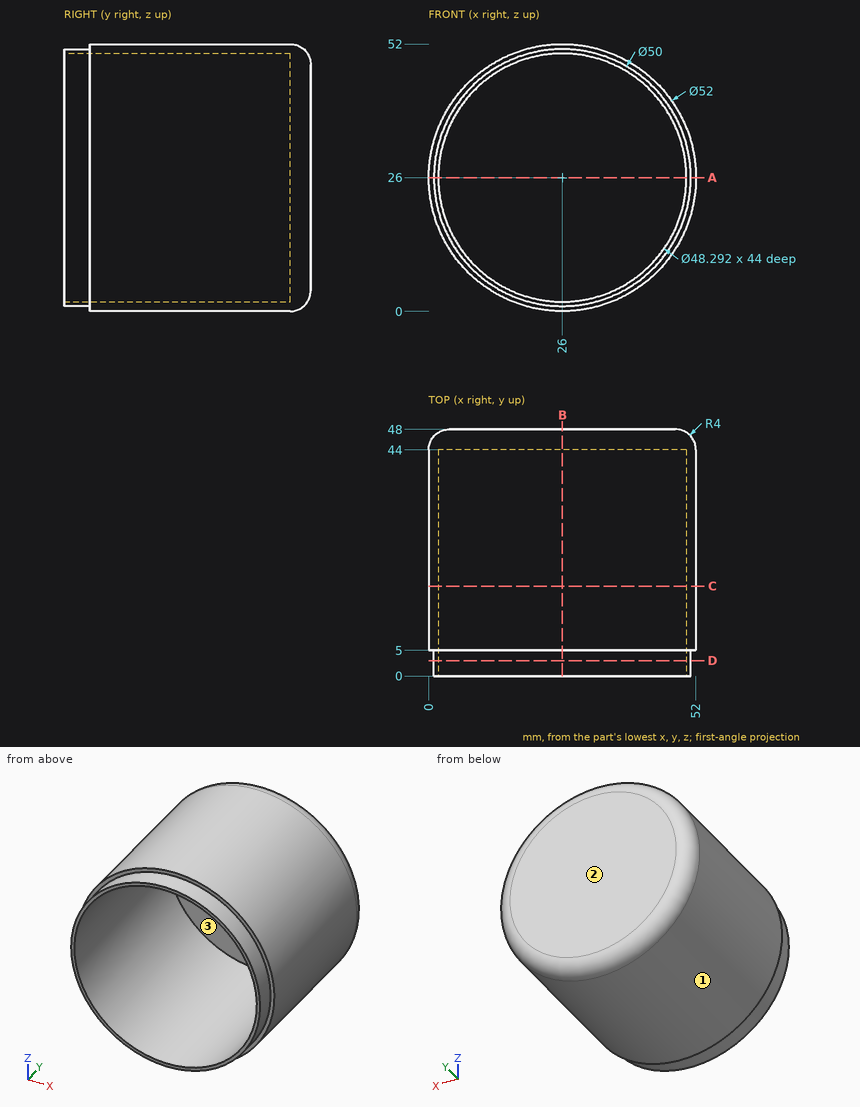
Geometry: see drawing. Coordinates: mm, zero at the bounding-box minimum. Coordinates: 2 decimals unless noted, no trailing zeros. Write each loop counter-clockwise with the first axis right and the second up, starting at its lowest first coordinate (ties: lowest second). Pieces come first, ordered by that corner, then holes. Notation, with made-up numbers: (76, 58) - (98, 58) arc R13 cw to (98, 71) - close; hole circle Ø4 at (3, 28.5). An arc over 180 degrees is marked (long way). Put each result on its own line as item: value. Start each with the question number.
1) Mould query, pull axis X, two halves, no side actions, for the marked faces 1, 2 and 3. Classes: pulls with the +X half, pulls with the -X half, needs draft (parallel to the pull), parting line crosses it, or undercut.
2) Cut plane A-A (z = 26). Return the cut outline in (x, y).
3) Cut plane B-B (x = 26). Return the cut outline in (y, z), plus the area to 3 significant figures.
4) Contact query for flat-ended pins moving along their axis: pin 1 (5 mm diameter, centred on y = 39.5, z = 7.5, fed in from -X); pin 2 (3 mm diameter, centred on x = 9.5, y = 34.5, fed in from +Z); pin 3 (5 mm diameter, centred on x = 42.5, y = 32.5, fed in from +Z). Output: stop coordinate, or through.
5) Cut plane D-D (y = 3). Return the cut outline in (x, z), plus the area to 3 significant figures.
6) Cut plane C-C (y = 17.5). Return the cut outline in (x, z), plus the area to 3 significant figures.
7) Ray query, L1, parallel to X at y = 33.5, z = 26; L2, parallel to Y at x = 11.5, z = 19.5; L3, parallel to X at y = 2, z = 6. Return the intervals inside material, ascending.
Resolved:
1. face 1: parting line crosses it
1. face 2: needs draft
1. face 3: undercut
2. outline: (0, 5) - (1, 5) - (1, 0) - (1.85, 0) - (1.85, 44) - (50.15, 44) - (50.15, 0) - (51, 0) - (51, 5) - (52, 5) - (52, 44) arc R4 ccw to (48, 48) - (4, 48) arc R4 ccw to (0, 44) - close
3. outline: (0, 1) - (5, 1) - (5, 0) - (44, 0) arc R4 ccw to (48, 4) - (48, 48) arc R4 ccw to (44, 52) - (5, 52) - (5, 51) - (0, 51) - (0, 50.15) - (44, 50.15) - (44, 1.85) - (0, 1.85) - close
3. area: 354 mm2
4. pin 1: stops at x = 5.51
4. pin 2: stops at z = 47.24
4. pin 3: stops at z = 47.91
5. outline: circle Ø50 at (26, 26); hole circle Ø48.29 at (26, 26)
5. area: 132 mm2
6. outline: circle Ø52 at (26, 26); hole circle Ø48.29 at (26, 26)
6. area: 292 mm2
7. L1: x = 0 to 1.85, 50.15 to 52
7. L2: y = 44 to 48
7. L3: x = 11 to 12.47, 39.53 to 41
